For this review, use the dimensioned drawing (mm, ordinates from the lowest corner) and the shaded views. Give positions to 0.01 mm unless a question says otherwise; leave off trailing zeros. Write each loop counter-clockwise with the first axis right and the second up, starting at its lowest first coordinate (ties: lowest second). Pieces come first, ordered by that corner, then holes.
1) We need section D-D on z = 21.5. Give the boundary of the cut face in (x, y), and give its area (3 significant figures).
2) We need section B-B on x = 12.5. Give the boundary of the cut face in (y, z), and give its area (3 significant figures).
3) Wall thickness on line 1 along X through (y, z) = (4.25, 12.5); line 2 along Y through (x, z) = (2.5, 18.5); line 3 along Z through (x, y) = (9.5, 5.7): over which ranges is each line inside the solid? List them lowest first.
4) For P1, Ø1, axis at x = 8, y = 4, coming from the -Z side; P2, Ø1.5, axis at y = 1.5, z = 3.5, coming from the +X side; P3, Ø3, axis at x = 18.5, y = 5, coming from the -Z side, all flat-tipped, find the tip position at first contact; note any pin that passes through.
5) Draft analysis for pull direction Z (two halves, no side actions). For the marked faces 1, 2 and 3, state which applies: pulls with the +Z half, pulls with the -Z half, needs draft (parallel to the pull), parting line crosses it, or undercut.
6) We need section A-A on z = 12.5. Give the boundary of the cut face in (x, y).
7) We need section C-C on y = 0.7. Give the boundary of the cut face in (x, z), and give its area (3 significant figures).
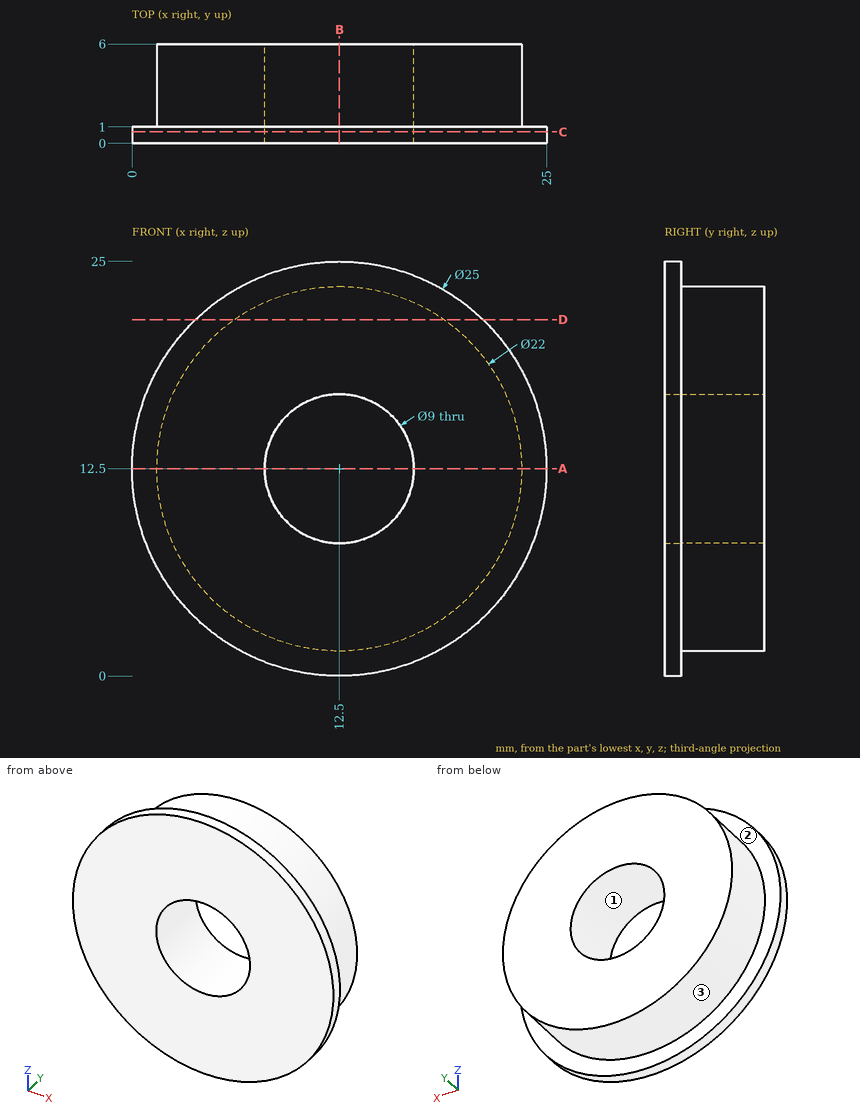
Results list:
1. outline: (3.83, 0) - (21.17, 0) - (21.17, 1) - (18.82, 1) - (18.82, 6) - (6.18, 6) - (6.18, 1) - (3.83, 1) - close
1. area: 80.6 mm2
2. outline: (0, 0) - (1, 0) - (1, 1.5) - (6, 1.5) - (6, 8) - (0, 8) - close; (0, 17) - (6, 17) - (6, 23.5) - (1, 23.5) - (1, 25) - (0, 25) - close
2. area: 81.0 mm2
3. line 1: x = 1.5 to 8, 17 to 23.5
3. line 2: y = 0 to 1
3. line 3: z = 1.92 to 9.15, 15.85 to 23.08
4. P1: stops at z = 2.25
4. P2: stops at x = 21.72
4. P3: stops at z = 2.46
5. face 1: undercut
5. face 2: needs draft
5. face 3: parting line crosses it
6. outline: (0, 0) - (8, 0) - (8, 6) - (1.5, 6) - (1.5, 1) - (0, 1) - close; (17, 0) - (25, 0) - (25, 1) - (23.5, 1) - (23.5, 6) - (17, 6) - close
7. outline: circle Ø25 at (12.5, 12.5); hole circle Ø9 at (12.5, 12.5)
7. area: 427 mm2
